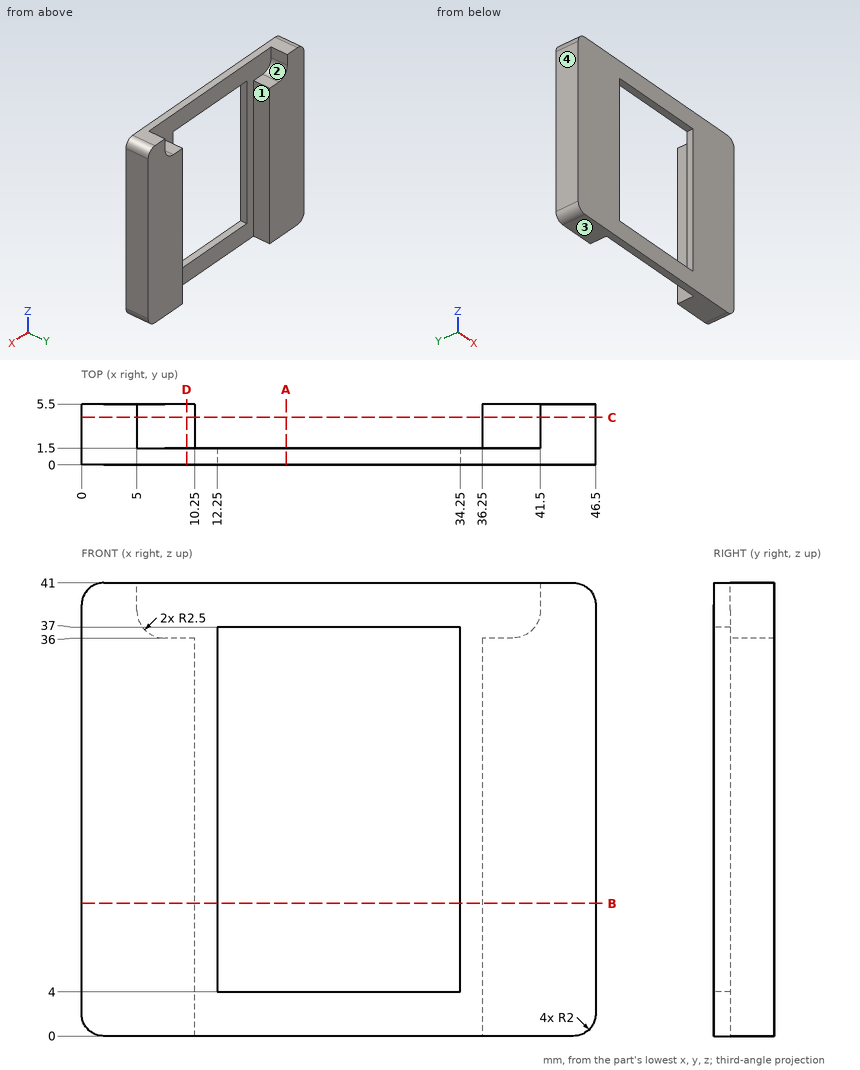
Study the drawing (mm; zero at the part's minimum x, y, z) and answer. Coordinates: 2 decimals unless noted, no trailing zeros. Write each loop counter-clockwise with the first axis right and the second up, starting at its lowest first coordinate (ties: lowest second). Pieces come first, ordered by that corner, then holes. Notation, with made-up numbers: M 20,-9 L 76,-9 A9 ccw 76,7 Z; hole C -16,45 d11. An arc over 180 degrees is marked long. Use one line per item in the form item = value.
Item 1: Find section C-C, the plane y = 4.3. Give the vertices of the cut face in (x, z), plus the area to 3 significant figures.
Model answer:
outline = M 0,2 A2 ccw 2,0 L 10.25,0 L 10.25,36 L 7.5,36 A2.5 cw 5,38.5 L 5,41 L 2,41 A2 ccw 0,39 Z; M 36.25,0 L 44.5,0 A2 ccw 46.5,2 L 46.5,39 A2 ccw 44.5,41 L 41.5,41 L 41.5,38.5 A2.5 cw 39,36 L 36.25,36 Z
area = 787 mm2
Item 2: Find the intervals of material crossed by probe 1 along X at (y, z) = (2.85, 20); probe 2 along X at (y, z) = (0.95, 16); probe 3 along Z at (x, y) = (27.5, 0.4), in increasing order.
Model answer:
probe_1 = 0 to 10.25, 36.25 to 46.5
probe_2 = 0 to 12.25, 34.25 to 46.5
probe_3 = 0 to 4, 37 to 41
Item 3: Find section B-B, the plane z = 12. Give the vertices of the cut face in (x, y), plus the area to 3 significant figures.
Model answer:
outline = M 0,0 L 12.25,0 L 12.25,1.5 L 10.25,1.5 L 10.25,5.5 L 0,5.5 Z; M 34.25,0 L 46.5,0 L 46.5,5.5 L 36.25,5.5 L 36.25,1.5 L 34.25,1.5 Z
area = 119 mm2
Item 4: Find section D-D, the plane x = 9.5. Give the vertices of the cut face in (y, z), plus the area to 4 significant figures.
Model answer:
outline = M 0,0 L 5.5,0 L 5.5,36 L 1.5,36 L 1.5,41 L 0,41 Z
area = 205.5 mm2
Item 5: Given P1, Ø2, axis at x = 9.5, y = 3, coming from the +Z side; P2, Ø8, axis at x = 27, z = 17.5, coming from the +Y side; P3, Ø0.8, axis at y = 3, z = 40.5, coming from the -X side; P4, Ø3, axis at x = 38, y = 3.5, coming from the +Z side, each flat-ended and moving along its own axis, determine where each tip first touches the part or whether it passes through.
Model answer:
P1 = 36
P2 = through
P3 = 0.33
P4 = 36.05
Item 6: Find section A-A, the plane x = 18.5. Give the vertices of the cut face in (y, z), plus the area to 3 significant figures.
Model answer:
outline = M 0,0 L 1.5,0 L 1.5,4 L 0,4 Z; M 0,37 L 1.5,37 L 1.5,41 L 0,41 Z
area = 12.0 mm2
Item 7: The mould has two halves that part along X. Classify the marked faces 1, 2, 3 and 4: released by +X, released by -X, zero draft, split by the parting line, or undercut.
Model answer:
face_1 = undercut
face_2 = undercut
face_3 = zero draft
face_4 = released by -X
